from build123d import *

# Parameters (mm, degrees)
RESSALTO_EXTRUS_O1_DEPTH = 2
ESBO_O2_R                = 1.5
CORTE_EXTRUS_O1_DEPTH    = 2


with BuildPart() as part:
    # Esboço1 → Ressalto-extrusão1 (new body)
    with BuildSketch(Plane.XY):
        with BuildLine():
            Line((-73.5, -27), (-73.5, 80))
            Line((-73.5, 80), (-38.5, 80))
            Line((-38.5, 80), (-38.5, 84))
            Line((-38.5, 84), (-73.5, 84))
            Line((-73.5, 84), (-73.5, 90))
            ThreePointArc((-73.5, 90), (-70.571067812, 97.071067812), (-63.5, 100))
            Line((-63.5, 100), (63.5, 100))
            ThreePointArc((63.5, 100), (70.571067812, 97.071067812), (73.5, 90))
            Line((73.5, 90), (73.5, 84))
            Line((73.5, 84), (38.5, 84))
            Line((38.5, 84), (38.5, 80))
            Line((38.5, 80), (73.5, 80))
            Line((73.5, 80), (73.5, -27))
            Line((73.5, -27), (38.5, -27))
            Line((38.5, -27), (38.5, -31))
            Line((38.5, -31), (73.5, -31))
            Line((73.5, -31), (73.5, -90))
            ThreePointArc((73.5, -90), (70.571067812, -97.071067812), (63.5, -100))
            Line((63.5, -100), (-63.5, -100))
            ThreePointArc((-63.5, -100), (-70.571067812, -97.071067812), (-73.5, -90))
            Line((-73.5, -90), (-73.5, -31))
            Line((-73.5, -31), (-38.5, -31))
            Line((-38.5, -31), (-38.5, -27))
            Line((-38.5, -27), (-73.5, -27))
        make_face()
    extrude(amount=RESSALTO_EXTRUS_O1_DEPTH)

    # Esboço2 → Corte-extrusão1 (cut)
    with BuildSketch(Plane.XY.offset(2)):
        with Locations((-52.5, 57)):
            Circle(ESBO_O2_R)
        with Locations((-52.5, 27)):
            Circle(ESBO_O2_R)
        with Locations((-52.5, 3)):
            Circle(ESBO_O2_R)
        with Locations((-52.5, -75)):
            Circle(ESBO_O2_R)
        with Locations((52.5, 57)):
            Circle(ESBO_O2_R)
        with Locations((52.5, -75)):
            Circle(ESBO_O2_R)
        with Locations((52.5, 3)):
            Circle(ESBO_O2_R)
        with Locations((52.5, 27)):
            Circle(ESBO_O2_R)
        with Locations((0, -75)):
            Circle(ESBO_O2_R)
    extrude(amount=-CORTE_EXTRUS_O1_DEPTH, mode=Mode.SUBTRACT)


solid = part.part
Geometry check sheet. Reference: the model listing, model coordinates, mm. Give positions to 0.01 mm unless a question says otherwise; leave off trailing zeros. Order: outer loops, then holes, each group sorted by start corner. A loop starts at its lowest first (then second) coordinate and runs counter-clockwise, first axis right, second up.
1) Material ranges on probe 1 along Y at (x, z) = (0, 0.7); probe 2 along X at (y, z) = (81.5, 0.9), recorded low to high.
Results are:
probe 1: y = -100 to -76.5, -73.5 to 100
probe 2: x = -38.5 to 38.5
2) Cross-section at B-B (z = 1). Give the number of separate pieces and of enclosed holes in the cut face, then the cut area to 3 significant figures.
Results are:
separate pieces: 1
enclosed holes: 9
area: 28,700 mm2
3) Gauge pin test, flat ends, axial feed: pin 1 (0.6 mm diameter, centred on y = 81, z = 1, fed in from -X); pin 2 (0.6 mm diameter, centred on y = 82, z = 0.5, fed in from +X); pin 3 (2.5 mm diameter, centred on x = 52.5, y = -75, fed in from +Z). Record the tip position at first contact, or that the pin passes through.
Results are:
pin 1: stops at x = -38.5
pin 2: stops at x = 38.5
pin 3: passes through
4) Cross-section at A-A (x = 59). Record the boundary of the cut face in (y, z).
Results are:
outline: (-100, 0) - (-31, 0) - (-31, 2) - (-100, 2) - close; (-27, 0) - (80, 0) - (80, 2) - (-27, 2) - close; (84, 0) - (100, 0) - (100, 2) - (84, 2) - close
